For this review, take the finished solid that the model builds, in its own axes (mm). A direction names the side the tool comes from. Round coordinates to 2 decimals unless told otherwise and drop trailing zeros. Order: outer loops, then holes, each group sorted by start corner. A loop starts at its lowest first (then second) coordinate and runs counter-clockwise, first axis right, second up. Notation, with made-up numbers: M 15.5,77 L 38.5,77 A13 ccw 38.5,87 Z; hole C 41.5,0.5 d1. An arc over 180 degrees is marked long. Answer as a JSON object with one key per item and string values.
from build123d import *

# Parameters (mm, degrees)
F0_R     = 12.5
F1_DEPTH = 0.625
F2_DEPTH = 1


with BuildPart() as f1:
    # F0 (on Top) → F1 (new body, symmetric)
    with BuildSketch(Plane.XY):
        Circle(F0_R)
        Polygon((-0.8784600757, 5.2192566285), (-0.8525428319, 5.1903319625), (0, 3.7833468732), (0.8525428319, 5.1903319625), (0.8784600757, 5.2192566285), (4.0636942722, 8.7741035968), (1.8921582399, 5.1903319625), (0.8525428319, 3.4746136163), (0.519807704, 2.9254877001), (6.4726816234, -6.8987751159), (5.7122610048, -7.3595412979), (0, 2.0676285271), (-5.7122610048, -7.3595412979), (-6.4726816234, -6.8987751159), (-0.519807704, 2.9254877001), (-0.8525428319, 3.4746136163), (-1.8921582399, 5.1903319625), (-4.0636942722, 8.7741035968), align=None, mode=Mode.SUBTRACT)
    extrude(amount=F1_DEPTH, both=True)

    # F0 (on Top) → F2 (join, symmetric)
    with BuildSketch(Plane.XY):
        Polygon((0, 3.7833468732), (-0.8525428319, 5.1903319625), (-0.8784600757, 5.2192566285), (-0.869668365, 5.1903319625), (-1.8921582399, 5.1903319625), (-0.8525428319, 3.4746136163), (-0.519807704, 2.9254877001), align=None)
        Polygon((0.8525428319, 5.1903319625), (0, 3.7833468732), (0.519807704, 2.9254877001), (0.8525428319, 3.4746136163), (1.8921582399, 5.1903319625), (0.869668365, 5.1903319625), (0.8784600757, 5.2192566285), align=None)
        Polygon((4.0636942722, 8.7741035968), (0.8784600757, 5.2192566285), (0.869668365, 5.1903319625), (1.8921582399, 5.1903319625), align=None)
        Polygon((-0.869668365, 5.1903319625), (-0.8784600757, 5.2192566285), (-4.0636942722, 8.7741035968), (-1.8921582399, 5.1903319625), align=None)
        Polygon((0.519807704, 2.9254877001), (0, 3.7833468732), (-0.519807704, 2.9254877001), (0, 2.0676285271), align=None)
        Polygon((0, 2.0676285271), (-0.519807704, 2.9254877001), (-6.4726816234, -6.8987751159), (-5.7122610048, -7.3595412979), align=None)
        Polygon((6.4726816234, -6.8987751159), (0.519807704, 2.9254877001), (0, 2.0676285271), (5.7122610048, -7.3595412979), align=None)
    extrude(amount=F2_DEPTH, both=True)


solid = f1.part
1) Mouldability with a two-part tool opening along X and no side actions: class faces 6 (the flat face through (-2.896, -2.712, -0.81)), 7 (the cylindrical face through (11.923, 3.755, 0.009)), 8 (the flat face through (3.54, -2.06, 0.82)) as +X half, -X half, draft (parallel to the pull), parting line (faces both ways), or undercut.
Geometry check:
{"face 6": "undercut", "face 7": "parting line", "face 8": "+X half"}
2) Add section B-B on x = -3.5. State the section outline as (y, z) points (3 decimals), and give its area (3 significant figures).
Geometry check:
{"outline": "M -12,-0.625 L -3.709,-0.625 L -3.709,-1 L -1.993,-1 L -1.993,-0.625 L 7.844,-0.625 L 7.844,-1 L 8.145,-1 L 8.145,-0.625 L 12,-0.625 L 12,0.625 L 8.145,0.625 L 8.145,1 L 7.844,1 L 7.844,0.625 L -1.993,0.625 L -1.993,1 L -3.709,1 L -3.709,0.625 L -12,0.625 Z", "area": "31.5 mm²"}
3) Insertion check: P1, Ø1, axis at y = -5, z = 0, coming from the +X side; P2, Ø1, axis at x = 9, y = 0.5, coming from the -Z side (3 decimals). Each pin has a flat end and moves straight along its axis. Give the tip position at first contact, or say it passes through.
Geometry check:
{"P1": "stops at x = 11.66", "P2": "stops at z = -0.625"}
4) Add section C-C on z = -0.25. State the section outline as (x, y) points, and give its area (3 significant figures).
Geometry check:
{"outline": "C 0,0 d25", "area": "491 mm²"}
5) For L1, parallel to Z at x = 4.5, y = -8 (3 decimals); L2, parallel to X at y = -4, z = 0.9; L3, parallel to X at y = -5, z = 0.75, list the stretches that pass through material, from the lowest coordinate up.
Geometry check:
{"L1": "z = -0.625 to 0.625", "L2": "x = -4.72 to -3.68, 3.68 to 4.72", "L3": "x = -5.32 to -4.28, 4.28 to 5.32"}
6) Machinability: for faces 1 (the flat face through (-3.455, -1.918, 0.815)), 2 (the flat face through (3.54, -2.06, -0.81)), 3 (the flat face through (0.432, 4.497, -0.81)), 4 (the flat face through (2.816, -2.58, 0.815)), 5 (the flat face through (-3.455, -1.918, -0.81)), which of the approach directions +Z, -Z, +X, -X, +Y, -Y give a long, thin tool a straight path to every point of the face, cutting with its end or side? Answer none if there is none.
Geometry check:
{"face 1": "+Z, -X", "face 2": "-Z, +X", "face 3": "-Z, +Y", "face 4": "+Z, -Y", "face 5": "-Z, -X"}
7) Add section D-D on x = 10. State the section outline as (y, z) points (3 decimals).
Geometry check:
{"outline": "M -7.5,-0.625 L 7.5,-0.625 L 7.5,0.625 L -7.5,0.625 Z"}
